```python
from build123d import *

# Parameters (mm, degrees)
REVOLVE1_ANGLE     = 180
SKETCH10_R         = 6
CUT_EXTRUDE1_DEPTH = 493.44289009


with BuildPart() as part:
    # Sketch1 → Revolve1 (revolve)
    with BuildSketch(Plane(origin=(0, 0, 0), x_dir=(1, 0, 0), z_dir=(0, 1, 0))):
        with BuildLine():
            Line((0, 250), (0, 243.75))
            ThreePointArc((0, 243.75), (-243.75, 0), (0, -243.75))
            Line((0, -243.75), (0, -250))
            ThreePointArc((0, -250), (-250, 0), (0, 250))
        make_face()
    revolve(axis=Axis((0, 0, -250), (0, 0, 1)), revolution_arc=REVOLVE1_ANGLE)

    # Sketch3 → Revolve2 (revolve)
    with BuildSketch(Plane(origin=(0, 0, 0), x_dir=(0, 0, -1), z_dir=(1, 0, 0)), mode=Mode.PRIVATE) as revolve2_sk:
        with BuildLine():
            Line((-250, 0), (-300, 0))
            Line((-300, 0), (-300, -12))
            Line((-300, -12), (-249.711833921, -12))
            ThreePointArc((-249.711833921, -12), (-249.927948097, -6.001729744), (-250, 0))
        make_face()
    revolve(revolve2_sk.sketch.rotate(Axis((0, 0, 0), (0, 1, 0)), 180), axis=Axis((0, 0, 0), (0, 1, 0)))

    # Sketch10 → Cut-Extrude1 (cut, through all)
    with BuildSketch(Plane(origin=(0, 0, 0), x_dir=(1, 0, 0), z_dir=(0, 1, 0))):
        with Locations(Location((0, 275, 0), (0, 0, 180))):
            Circle(SKETCH10_R)
        with Locations(Location((-137.5, 238.156986041, 0), (0, 0, 180))):
            Circle(SKETCH10_R)
        with Locations(Location((-238.156986041, 137.5, 0), (0, 0, 180))):
            Circle(SKETCH10_R)
        with Locations(Location((-275, 0, 0), (0, 0, 180))):
            Circle(SKETCH10_R)
        with Locations(Location((-238.156986041, -137.5, 0), (0, 0, 180))):
            Circle(SKETCH10_R)
        with Locations(Location((-137.5, -238.156986041, 0), (0, 0, 180))):
            Circle(SKETCH10_R)
        with Locations(Location((0, -275, 0), (0, 0, 180))):
            Circle(SKETCH10_R)
        with Locations(Location((137.5, -238.156986041, 0), (0, 0, 180))):
            Circle(SKETCH10_R)
        with Locations(Location((238.156986041, -137.5, 0), (0, 0, 180))):
            Circle(SKETCH10_R)
        with Locations(Location((275, 0, 0), (0, 0, 180))):
            Circle(SKETCH10_R)
        with Locations(Location((238.156986041, 137.5, 0), (0, 0, 180))):
            Circle(SKETCH10_R)
        with Locations(Location((137.5, 238.156986041, 0), (0, 0, 180))):
            Circle(SKETCH10_R)
    extrude(amount=-CUT_EXTRUDE1_DEPTH, mode=Mode.SUBTRACT)


solid = part.part
```
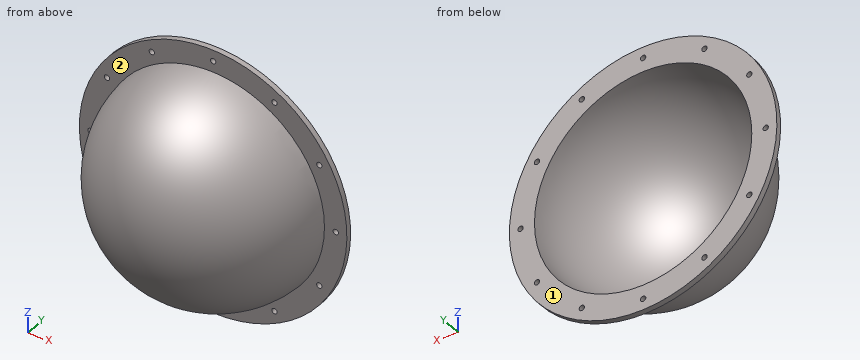
Source: CAD feature listing. Evaluate the final solid. Frame: model axes, mm. Face numbers are marked on the shaded views. A direction names the side the tool comes from. Coordinates: 2 decimals unless noted, no trailing zeros. Loops run counter-clockwise (first coordinate to the right, second up) from the corner with the lowest first, then second, coordinate; pieces in that order, holes last. Notation, with made-up numbers: (11.5, -5) -> (60.5, -5) arc R18 cw to (60.5, 21) -> close; hole circle Ø10 at (17, -0.5). An arc over 180 degrees is marked (long way). One line per item, written item: value. Start each with the question number.
Q1. Set-up query: the marked faces 1 and 2. Return all of +Z, -Z, +X, -X, +Y, -Y with unobstructed straight access to the full face (end or side cutting, diameter ignored); none if empty.
Q2. Contact query for flat-ended pins moving along their axis: P1, Ø14, axis at x = 0, z = -275, coming from the -Y side; P2, Ø4, axis at x = 63, z = 153.5, coming from the -Y side (3 decimals); P3, Ø5, axis at x = 88, y = -153, coming from the +Z side. Output: stop coordinate, or through.
Q3. Section query A-A, the plane z = -183. Return the cut outline in (x, y), and give its area (3 significant figures).
Q4. Line query: line 1 along X through (y, z) = (-6, -137); line 2 along X through (y, z) = (-62, -29); line 3 along X through (y, z) = (-171, -137). Output: solid intervals per line, ascending.
Q5. Section query B-B, the plane x = 164.5. Return the cut outline in (y, z), and give its area (3 significant figures).
Q6. Section query C-C, the plane y = -212. Return the cut outline in (x, z).
Results:
1. face 1: +Z, -Z, +X, -X, +Y
1. face 2: -Y
2. P1: y = -12
2. P2: y = -188.755
2. P3: z = 179.51
3. outline: (-237.72, -12) -> (-169.9, -12) arc R170.33 ccw to (169.9, -12) -> (237.72, -12) -> (237.72, 0) -> (161.01, 0) arc R161.01 cw to (-161.01, 0) -> (-237.72, 0) -> close
3. area: 6,470 mm^2
4. line 1: -266.89 to -244.14, -232.18 to -201.52, 201.52 to 232.18, 244.14 to 266.89
4. line 2: -240.45 to -233.94, 233.94 to 240.45
4. line 3: -120.37 to -106.79, 106.79 to 120.37
5. outline: (-12, -250.88) -> (0, -250.88) -> (0, -179.87) arc R179.87 cw to (0, 179.87) -> (0, 250.88) -> (-12, 250.88) -> (-12, 187.87) arc R188.25 ccw to (-12, -187.87) -> close
5. area: 6,350 mm^2
6. outline: circle Ø265 at (0, 0); hole circle Ø240.58 at (0, 0)
